```python
from build123d import *

# Parameters (mm, degrees)
SKETCH1_W           = 1.5
SKETCH1_H           = 152.24
SKETCH2_R           = 16.75
BOSS_EXTRUDE1_DEPTH = 2.14
SKETCH4_R           = 15
BOSS_EXTRUDE2_DEPTH = 2.14


with BuildPart() as part:
    # Sketch1 → Revolve1 (revolve)
    with BuildSketch(Plane.XY):
        with Locations((13.565, 76.12)):
            Rectangle(SKETCH1_W, SKETCH1_H)
    revolve(axis=Axis((0, 0, 0), (0, 1, 0)))

    # Sketch2 → Boss-Extrude1 (add)
    with BuildSketch(Plane(origin=(0, 0, 0), x_dir=(1, 0, 0), z_dir=(0, 1, 0))):
        Circle(SKETCH2_R)
    extrude(amount=BOSS_EXTRUDE1_DEPTH)

    # Sketch4 → Boss-Extrude2 (add)
    with BuildSketch(Plane(origin=(0, 2.14, 0), x_dir=(1, 0, 0), z_dir=(0, 1, 0))):
        Circle(SKETCH4_R)
    extrude(amount=BOSS_EXTRUDE2_DEPTH)


solid = part.part
```
Build history of the part. All positions in model axes, mm. A direction names the side the tool comes from. Round coordinates to 2 decimals unless told otherwise and drop trailing zeros. Write each loop counter-clockwise with the first axis right and the second up, starting at its lowest first coordinate (ties: lowest second). Pieces come first, ordered by that corner, then holes. Notation, with made-up numbers: (70.5, 16.25) -> (79.5, 16.25) arc R17 cw to (79.5, 43.25) -> close; hole circle Ø7 at (66, -31). An arc over 180 degrees is marked (long way). Put each result on its own line as item: value.
Item 1: Tool access for faces 5 (the face through (-3.63, 1.06, 16.35)), 6 (the face through (-12.5, 2.14, 8.6)): list every direction of +Z, -Z, +X, -X, +Y, -Y with a clear straight run to the whole face (end or side of a thin tool).
Here are the results:
face 5: +Y, -Y
face 6: +Y
Item 2: Flat gauge pins, fed straight in: P1, Ø3, axis at y = 58, z = -12, coming from the +X side; P2, Ø4, axis at y = 72, z = -13, coming from the -X side; P3, Ø4, axis at x = 7.5, y = 56, coming from the -Z side. Where does each tip first touch, or does it go through?
Here are the results:
P1: stops at x = 9.73
P2: stops at x = -9.16
P3: stops at z = -13.22
Item 3: Slice it at B-B, the plane x = 0. Give the cut face in (y, z) (3 decimals), plus the area to 3 significant figures.
Here are the results:
outline: (0, -16.75) -> (2.14, -16.75) -> (2.14, -15) -> (4.28, -15) -> (4.28, -14.315) -> (152.24, -14.315) -> (152.24, -12.815) -> (4.28, -12.815) -> (4.28, 12.815) -> (152.24, 12.815) -> (152.24, 14.315) -> (4.28, 14.315) -> (4.28, 15) -> (2.14, 15) -> (2.14, 16.75) -> (0, 16.75) -> close
area: 580 mm^2
Item 4: Wall check: probe 1 along X at (y, z) = (97, 0) (3 decimals); probe 2 along Y at (x, z) = (-7, -4). Give the ranges that are in metal, low to high. Write a range as from..to.
Here are the results:
probe 1: x = -14.315..-12.815, 12.815..14.315
probe 2: y = 0..4.28
Item 5: Slice it at C-C, the plane y = 66.5. Give the cut face in (x, z) (3 decimals), plus the area to 3 significant figures.
Here are the results:
outline: circle Ø28.63 at (0, 0); hole circle Ø25.63 at (0, 0)
area: 128 mm^2
Item 6: Two-plate mould, pull along Z, no slides. Class faces 1 (the face through (-9.445, 79.296, -8.661)), 2 (the face through (-14.985, 3.195, -0.66)), 3 (the face through (0, 4.28, 0)), 4 (the face through (11, 152.24, 7)): pulls with the +Z half, pulls with the -Z half, needs draft (parallel to the pull), parting line crosses it, or undercut.
Here are the results:
face 1: undercut
face 2: parting line crosses it
face 3: undercut
face 4: needs draft
Item 7: Slice it at A-A, the plane z = 0. Give the cut face in (x, y) (3 decimals), plus the area to 3 significant figures.
Here are the results:
outline: (-16.75, 0) -> (16.75, 0) -> (16.75, 2.14) -> (15, 2.14) -> (15, 4.28) -> (14.315, 4.28) -> (14.315, 152.24) -> (12.815, 152.24) -> (12.815, 4.28) -> (-12.815, 4.28) -> (-12.815, 152.24) -> (-14.315, 152.24) -> (-14.315, 4.28) -> (-15, 4.28) -> (-15, 2.14) -> (-16.75, 2.14) -> close
area: 580 mm^2
